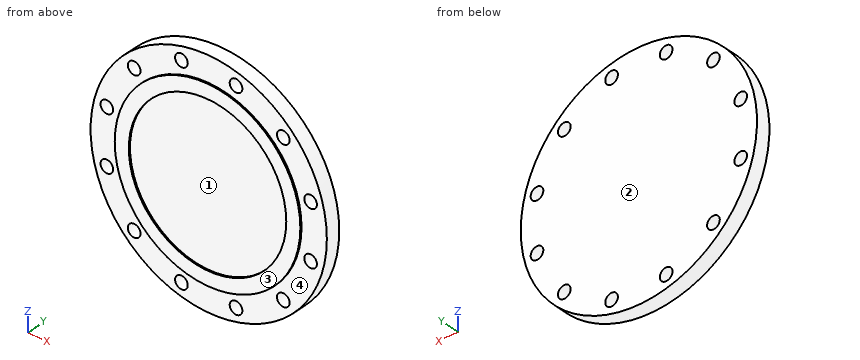
```python
from build123d import *

# Parameters (mm, degrees)
F0_R     = 266.7
F0_R_2   = 14.2875
F0_R_3   = 177.8
F1_DEPTH = 33.274
F2_R     = 209.55
F2_R_2   = 177.8
F3_DEPTH = 3.175
F4_R     = 177.8
F5_DEPTH = 33.274


with BuildPart() as f1:
    # F0 (on Front) → F1 (new body)
    with BuildSketch(Plane.XZ):
        Circle(F0_R)
        with Locations((-168.379802, -168.379802)):
            Circle(F0_R_2, mode=Mode.SUBTRACT)
        with Locations((-61.631285, -230.011087)):
            Circle(F0_R_2, mode=Mode.SUBTRACT)
        with Locations((-230.011087, -61.631285)):
            Circle(F0_R_2, mode=Mode.SUBTRACT)
        with Locations((61.631285, -230.011087)):
            Circle(F0_R_2, mode=Mode.SUBTRACT)
        with Locations((168.379802, -168.379802)):
            Circle(F0_R_2, mode=Mode.SUBTRACT)
        with Locations((230.011087, -61.631285)):
            Circle(F0_R_2, mode=Mode.SUBTRACT)
        with Locations((-230.011087, 61.631285)):
            Circle(F0_R_2, mode=Mode.SUBTRACT)
        with Locations((-168.379802, 168.379802)):
            Circle(F0_R_2, mode=Mode.SUBTRACT)
        with Locations((-61.631285, 230.011087)):
            Circle(F0_R_2, mode=Mode.SUBTRACT)
        Circle(F0_R_3, mode=Mode.SUBTRACT)
        with Locations((230.011087, 61.631285)):
            Circle(F0_R_2, mode=Mode.SUBTRACT)
        with Locations((61.631285, 230.011087)):
            Circle(F0_R_2, mode=Mode.SUBTRACT)
        with Locations((168.379802, 168.379802)):
            Circle(F0_R_2, mode=Mode.SUBTRACT)
    extrude(amount=F1_DEPTH)

    # F2 (on face) → F3 (join)
    with BuildSketch(Plane.XZ.offset(33.274)):
        Circle(F2_R)
        Circle(F2_R_2, mode=Mode.SUBTRACT)
    extrude(amount=F3_DEPTH)

    # F4 (on face) → F5 (join)
    with BuildSketch(Plane.XZ.offset(33.274)):
        Circle(F4_R)
    extrude(amount=-F5_DEPTH)


solid = f1.part
```
Verification items for the finished model (mm, model axes). Face numbers are marked on the shaded views. A direction names the side the tool comes from. Round coordinates to 2 decimals unless told otherwise and drop trailing zeros. Order: outer loops, then holes, each group sorted by start corner. A loop starts at its lowest first (then second) coordinate and runs counter-clockwise, first axis right, second up. Notation, with made-up numbers: (59.25, -23.75) -> (82.25, -23.75) arc R7 ccw to (82.25, -12.75) -> close; hole circle Ø4 at (3.25, 68). An arc over 180 degrees is marked (long way). Put each result on its own line as item: value. Start each with the question number.
(1) Section check C-C (x = 0). Enter the section's corners in (y, z).
(2) Draft check along X on the marked faces 1 and 2. Enter one of: +X half, -X half, draft (parallel to the pull), parting line (faces both ways), or undercut.
(3) Section check B-B (z = 0). Enter the section's corners in (x, y), then the cut area to 4 significant figures.
(4) Material ranges on line 1 along Z through (x, y) = (-243, -32); line 2 along X through (y, z) = (-26.5, 63); line 3 along X through (y, z) = (-29, 239), recorded low to high.
(5) Section check A-A (x = -169.5). Enter the section's corners in (y, z), then the cut area to 3 significant figures.
(6) Section check D-D (x = -57.5). Enter the section's corners in (y, z), then the cut area to 3 significant figures.
(7) Tool access check on the marked faces 3 and 4. Record the directions out of +Z, -Z, +X, -X, +Y, -Y that give a thin tool (end or side, any length) a straight path to the whole face; none if there is none.
(8) Depth check by flat-ended pin: pin 1 Ø6 at (x, y) = (-190.5, -19.5) entering from +Z; pin 2 Ø8 at (y, z) = (-31.5, 140) entering from +X; pin 3 Ø12 at (y, z) = (-14, 130) entering from +X; pin 4 Ø17 at (x, z) = (-61.63, 230.01) entering from +Y. Enter the tip coordinate at first touch or a pass-through.
Completed:
1. outline: (-36.45, -209.55) -> (-33.27, -209.55) -> (-33.27, -266.7) -> (0, -266.7) -> (0, 266.7) -> (-33.27, 266.7) -> (-33.27, 209.55) -> (-36.45, 209.55) -> (-36.45, 177.8) -> (-33.27, 177.8) -> (-33.27, -177.8) -> (-36.45, -177.8) -> close
2. face 1: undercut
2. face 2: draft
3. outline: (-266.7, -33.27) -> (-209.55, -33.27) -> (-209.55, -36.45) -> (-177.8, -36.45) -> (-177.8, -33.27) -> (177.8, -33.27) -> (177.8, -36.45) -> (209.55, -36.45) -> (209.55, -33.27) -> (266.7, -33.27) -> (266.7, 0) -> (-266.7, 0) -> close
3. area: 17,950 mm2
4. line 1: z = -109.91 to -67.58, -55.68 to 55.68, 67.58 to 109.91
4. line 2: x = -259.15 to -244.23, -215.79 to 215.79, 244.23 to 259.15
4. line 3: x = -118.35 to -72.74, -50.53 to 50.53, 72.74 to 118.35
5. outline: (-36.45, -123.21) -> (-33.27, -123.21) -> (-33.27, -154.14) -> (0, -154.14) -> (0, 154.14) -> (-33.27, 154.14) -> (-33.27, 123.21) -> (-36.45, 123.21) -> (-36.45, 53.69) -> (-33.27, 53.69) -> (-33.27, -53.69) -> (-36.45, -53.69) -> close; (-33.27, -205.91) -> (0, -205.91) -> (0, -182.62) -> (-33.27, -182.62) -> close; (-33.27, 182.62) -> (0, 182.62) -> (0, 205.91) -> (-33.27, 205.91) -> close
5. area: 12,200 mm2
6. outline: (-36.45, -201.51) -> (-33.27, -201.51) -> (-33.27, -216.33) -> (0, -216.33) -> (0, 216.33) -> (-33.27, 216.33) -> (-33.27, 201.51) -> (-36.45, 201.51) -> (-36.45, 168.25) -> (-33.27, 168.25) -> (-33.27, -168.25) -> (-36.45, -168.25) -> close; (-33.27, -260.43) -> (0, -260.43) -> (0, -243.69) -> (-33.27, -243.69) -> close; (-33.27, 243.69) -> (0, 243.69) -> (0, 260.43) -> (-33.27, 260.43) -> close
6. area: 15,700 mm2
7. face 3: +Z, -Z, +X, -X, -Y
7. face 4: -Y
8. pin 1: stops at z = 189.66
8. pin 2: stops at x = 229.42
8. pin 3: stops at x = 236.12
8. pin 4: passes through
